```python
from build123d import *

# Parameters (mm, degrees)
SKETCH2_W           = 57.15
SKETCH2_H           = 49.784
BOSS_EXTRUDE1_DEPTH = 14.224
SKETCH3_W           = 44.196
SKETCH3_H           = 39.37
CUT_EXTRUDE1_DEPTH  = 8.255
SKETCH4_W           = 35.56
SKETCH4_H           = 4.191
SKETCH4_W_2         = 15.621
SKETCH4_H_2         = 6.858
CUT_EXTRUDE2_DEPTH  = 8.255
SKETCH5_W           = 7.62
SKETCH5_H           = 8.89
SKETCH5_H_2         = 7.62
BOSS_EXTRUDE2_DEPTH = 6.604
SKETCH6_W           = 2.54
SKETCH6_H           = 5.08
SKETCH6_W_2         = 5.08
SKETCH6_H_2         = 2.54
CUT_EXTRUDE3_DEPTH  = 6.604
FILLET1_R           = 5.08
FILLET2_R           = 2.54
SKETCH7_W           = 76.2
SKETCH7_H           = 14.224
SKETCH7_R           = 2.38125
BOSS_EXTRUDE3_DEPTH = 5.207
BOSS_EXTRUDE4_DEPTH = 76.2
SKETCH9_R           = 2.413
CUT_EXTRUDE4_DEPTH  = 25.4
CHAMFER1_SIZE       = 5.08
CHAMFER1_SIZE_2     = 8.798818102
CHAMFER2_SIZE       = 5.08
CHAMFER2_SIZE_2     = 8.798818102
FILLET3_R           = 5.08
FILLET4_R           = 5.08


# Some blends are built 0.0001 mm under size
with BuildPart() as part:
    # Sketch2 → Boss-Extrude1 (new body)
    with BuildSketch(Plane(origin=(0, 0, 0), x_dir=(1, 0, 0), z_dir=(0, 1, 0))):
        with Locations((28.575, 24.892)):
            Rectangle(SKETCH2_W, SKETCH2_H)
    extrude(amount=BOSS_EXTRUDE1_DEPTH)

    # Sketch3 → Cut-Extrude1 (cut)
    with BuildSketch(Plane(origin=(0, 14.224, 0), x_dir=(1, 0, 0), z_dir=(0, 1, 0))):
        with Locations((28.575, 24.892)):
            Rectangle(SKETCH3_W, SKETCH3_H)
    extrude(amount=-CUT_EXTRUDE1_DEPTH, mode=Mode.SUBTRACT)

    # Sketch4 → Cut-Extrude2 (cut)
    with BuildSketch(Plane(origin=(0, 5.969, 0), x_dir=(1, 0, 0), z_dir=(0, 1, 0))):
        with Locations((28.575, 12.5095)):
            Rectangle(SKETCH4_W, SKETCH4_H)
        with Locations((28.575, 24.638)):
            Rectangle(SKETCH4_W_2, SKETCH4_H_2)
    extrude(amount=-CUT_EXTRUDE2_DEPTH, mode=Mode.SUBTRACT)

    # Sketch5 → Boss-Extrude2 (add)
    with BuildSketch(Plane(origin=(0, 14.224, 0), x_dir=(1, 0, 0), z_dir=(0, 1, 0))):
        with Locations((-3.81, 24.765)):
            Rectangle(SKETCH5_W, SKETCH5_H)
        Polygon((12.7, 49.784), (36.83, 49.784), (44.45, 49.784), (44.45, 57.404), (36.83, 57.404), (12.7, 57.404), align=None)
        with Locations((60.96, 24.765)):
            Rectangle(SKETCH5_W, SKETCH5_H_2)
    extrude(amount=-BOSS_EXTRUDE2_DEPTH)

    # Sketch6 → Cut-Extrude3 (cut)
    with BuildSketch(Plane(origin=(0, 14.224, 0), x_dir=(1, 0, 0), z_dir=(0, 1, 0))):
        with Locations((-3.81, 24.765)):
            Rectangle(SKETCH6_W, SKETCH6_H)
        with Locations((60.96, 24.765)):
            Rectangle(SKETCH6_W, SKETCH6_H)
        with Locations((16.51, 53.594)):
            Rectangle(SKETCH6_W_2, SKETCH6_H_2)
        with Locations((40.64, 53.594)):
            Rectangle(SKETCH6_W_2, SKETCH6_H_2)
    extrude(amount=-CUT_EXTRUDE3_DEPTH, mode=Mode.SUBTRACT)

    # Fillet1
    fillet1_edges = [part.edges().sort_by_distance(p)[0] for p in [
        (0, 7.112, -49.784),
        (57.15, 7.112, -49.784),
        (57.15, 7.112, 0),
        (0, 7.112, 0),
    ]]
    fillet(fillet1_edges, radius=FILLET1_R)

    # Fillet2
    fillet2_edges = [part.edges().sort_by_distance(p)[0] for p in [
        (-7.62, 10.922, -20.32),
        (-7.62, 10.922, -29.21),
        (12.7, 10.922, -57.404),
        (44.45, 10.922, -57.404),
        (64.77, 10.922, -28.575),
        (64.77, 10.922, -20.955),
    ]]
    fillet(fillet2_edges, radius=FILLET2_R)

    # Sketch7 → Boss-Extrude3 (add)
    with BuildSketch(Plane.XY):
        with Locations((28.575, 7.112)):
            Rectangle(SKETCH7_W, SKETCH7_H)
        with Locations((-5.461, 7.112)):
            Circle(SKETCH7_R, mode=Mode.SUBTRACT)
        with Locations((62.611, 7.112)):
            Circle(SKETCH7_R, mode=Mode.SUBTRACT)
    extrude(amount=-BOSS_EXTRUDE3_DEPTH)

    # Sketch8 → Boss-Extrude4 (add)
    with BuildSketch(Plane.ZY.offset(9.525)):
        Polygon((-5.207, 0), (-5.207, 14.224), (8.212230229, 14.224), (0, 0), align=None)
    extrude(amount=-BOSS_EXTRUDE4_DEPTH)

    # Sketch9 → Cut-Extrude4 (cut)
    with BuildSketch(Plane(origin=(0, 0, 0), x_dir=(1, 0, 0), z_dir=(0, -0.5000000000000043, 0.8660254037844363))):
        with Locations(Location((-4.699, 6.264460458, 0), (0, 0, 270))):
            Circle(SKETCH9_R)
        with Locations(Location((61.849, 6.264460458, 0), (0, 0, 270))):
            Circle(SKETCH9_R)
    extrude(amount=-CUT_EXTRUDE4_DEPTH, mode=Mode.SUBTRACT)

    # Chamfer1
    # the kernel refuses this chamfer: 8.798818102, 5.08 mm, written as the material it takes off along each edge
    with BuildSketch(Plane(origin=(57.15, 14.224, -5.207), x_dir=(0, 0.05789386240267539, 0.9983227437537924), z_dir=(1, 0, 0))) as chamfer1_piece_1:
        Polygon((CHAMFER1_SIZE * 0.998322743754, CHAMFER1_SIZE * 0.0578938624027), (-CHAMFER1_SIZE_2 * 0.0578938624056, CHAMFER1_SIZE_2 * 0.998322743805), (0, 0), align=None)
    extrude(amount=32.288296971, mode=Mode.SUBTRACT)

    # Chamfer2
    # the kernel refuses this chamfer: 8.798818102, 5.08 mm, written as the material it takes off along each edge
    with BuildSketch(Plane(origin=(-32.288296971, 14.224, -5.207), x_dir=(0, 0.05789386240267139, 0.9983227437537925), z_dir=(1, 0, 0))) as chamfer2_piece_1:
        Polygon((CHAMFER2_SIZE * 0.998322743754, CHAMFER2_SIZE * 0.0578938624027), (-CHAMFER2_SIZE_2 * 0.0578938624056, CHAMFER2_SIZE_2 * 0.998322743805), (0, 0), align=None)
    extrude(amount=32.288296971, mode=Mode.SUBTRACT)

    # Fillet3
    fillet3_edges = [part.edges().sort_by_distance(p)[0] for p in [
        (44.45, 10.922, -49.784),
        (12.7, 10.922, -49.784),
    ]]
    fillet(fillet3_edges, radius=FILLET3_R - 0.0001)  # a hair under: the kernel refuses the full size

    # Fillet4
    fillet4_edges = [part.edges().sort_by_distance(p)[0] for p in [
        (57.15, 10.922, -20.955),
        (57.15, 10.922, -28.575),
        (0, 10.922, -29.21),
        (0, 10.922, -20.32),
    ]]
    fillet(fillet4_edges, radius=FILLET4_R - 0.0001)  # a hair under: the kernel refuses the full size


solid = part.part
```
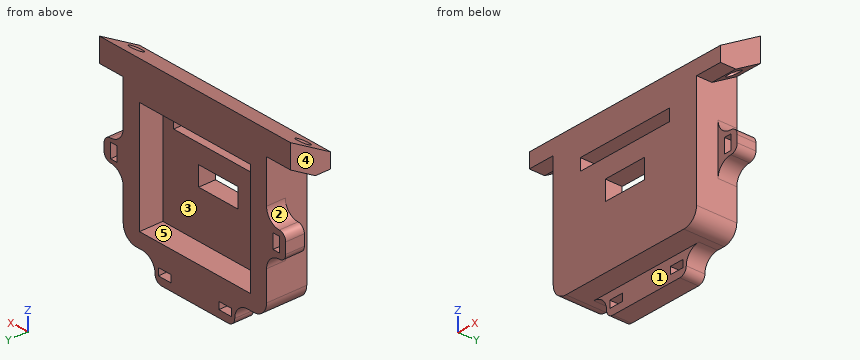
For this review, take the finished solid that the model builds, in its own axes (mm). Face numbers are marked on the shaded views. A direction names the side the tool comes from. Coordinates: 2 decimals unless noted, no trailing zeros. Order: outer loops, then holes, each group sorted by start corner. A loop starts at its lowest first (then second) coordinate and runs counter-clockwise, first axis right, second up. Notation, with made-up numbers: (75.25, -24.75) -> (86.25, -24.75) arc R24 ccw to (86.25, 2.25) -> close; hole circle Ø8 at (36, -36.75). An arc over 180 degrees is marked (long way). Use CSV: the item, a comma, the result in double quotes. Start each with the question number.
Item 1: For the marked faces 4 and 5, list the 3-axis set-ups (+Z, -Z, +X, -X, +Y, -Y) from which the entire face can be reached by the end or side of a thin tool; tool diameter is ignored.
Item 2: We need section C-C, the plane y = 1. Give the number of separate pieces and of enclosed holes in the cut face, then the cut area to 3 significant figures.
Item 3: We need section D-D, the plane x = 9. Give the boundary of the cut face in (y, z) (3 decimals), then the cut area to 3 significant figures.
Item 4: Wall thickness on probe 1 along X at (y, z) = (13.25, -25); probe 2 along X at (y, z) = (10.5, -9.5); probe 3 along X at (y, z) = (1.5, -10.5) (3 decimals): over which ranges is each line inside the solid? List them lowest first.
Item 5: Insertion check: pin 1 (1.3 mm diameter, centred on y = 11.5, z = -54, fed in from +X); pin 2 (2.5 mm diameter, centred on y = 10.5, z = -25.5, fed in from +X); pin 3 (12 mm diameter, centred on x = 37.5, z = -22.5, fed in from +Y). Each pin has a flat end and moves straight along its axis. Give the tip position at first contact, or say it passes through.
Item 6: Draft analysis for pull direction X (two halves, no side actions). For the marked faces 1, 2 and 3, state which applies: pulls with the +X half, pulls with the -X half, needs draft (parallel to the pull), parting line crosses it, or undercut.
Item 7: We need section B-B, the plane z = -24.5. Give the boundary of the cut face in (x, y), then the cut area to 3 significant figures.
Item 8: We need section A-A, the plane x = 24.5. Give the boundary of the cut face in (y, z) (3 decimals), then the cut area to 3 significant figures.
Derived:
1,face 4,"+Z, -Z, -X, +Y, -Y"
1,face 5,"+Y"
2,separate pieces,"1"
2,enclosed holes,"2"
2,area,"2,720 mm^2"
3,outline,"(0, -49.784) -> (7.62, -49.784) -> (7.62, -49.975) -> (14.224, -49.975) -> (14.224, -44.577) -> (5.969, -44.577) -> (5.969, -5.207) -> (14.224, -5.207) -> (14.224, 8.212) -> (0, 0) -> close"
3,area,"443 mm^2"
4,probe 1,"x = -7.62 to -5.08, -2.54 to 6.48, 50.67 to 59.69, 62.23 to 64.77"
4,probe 2,"x = 0 to 6.48, 50.67 to 57.15"
4,probe 3,"x = 0 to 10.795, 46.355 to 57.15"
5,pin 1,"stops at x = 44.68"
5,pin 2,"stops at x = 64.77"
5,pin 3,"stops at y = 5.97"
6,face 1,"needs draft"
6,face 2,"pulls with the -X half"
6,face 3,"undercut"
7,outline,"(-7.62, 7.62) -> (-5.08, 7.62) -> (-5.08, 14.22) -> (-7.62, 14.22) -> close; (-2.54, 7.62) -> (0, 7.62) -> (0, 0) -> (20.76, 0) -> (20.76, 5.97) -> (6.48, 5.97) -> (6.48, 14.22) -> (-2.54, 14.22) -> close; (36.39, 0) -> (57.15, 0) -> (57.15, 7.62) -> (59.69, 7.62) -> (59.69, 14.22) -> (50.67, 14.22) -> (50.67, 5.97) -> (36.39, 5.97) -> close; (62.23, 7.62) -> (64.77, 7.62) -> (64.77, 14.22) -> (62.23, 14.22) -> close"
7,area,"422 mm^2"
8,outline,"(0, -49.784) -> (7.62, -49.784) -> (7.62, -57.404) -> (14.224, -57.404) -> (14.224, -44.577) -> (5.969, -44.577) -> (5.969, -28.067) -> (0, -28.067) -> close; (0, -21.209) -> (5.969, -21.209) -> (5.969, -14.605) -> (0, -14.605) -> close; (0, -10.414) -> (5.969, -10.414) -> (5.969, -5.207) -> (14.224, -5.207) -> (14.224, 8.212) -> (0, 0) -> close"
8,area,"426 mm^2"
